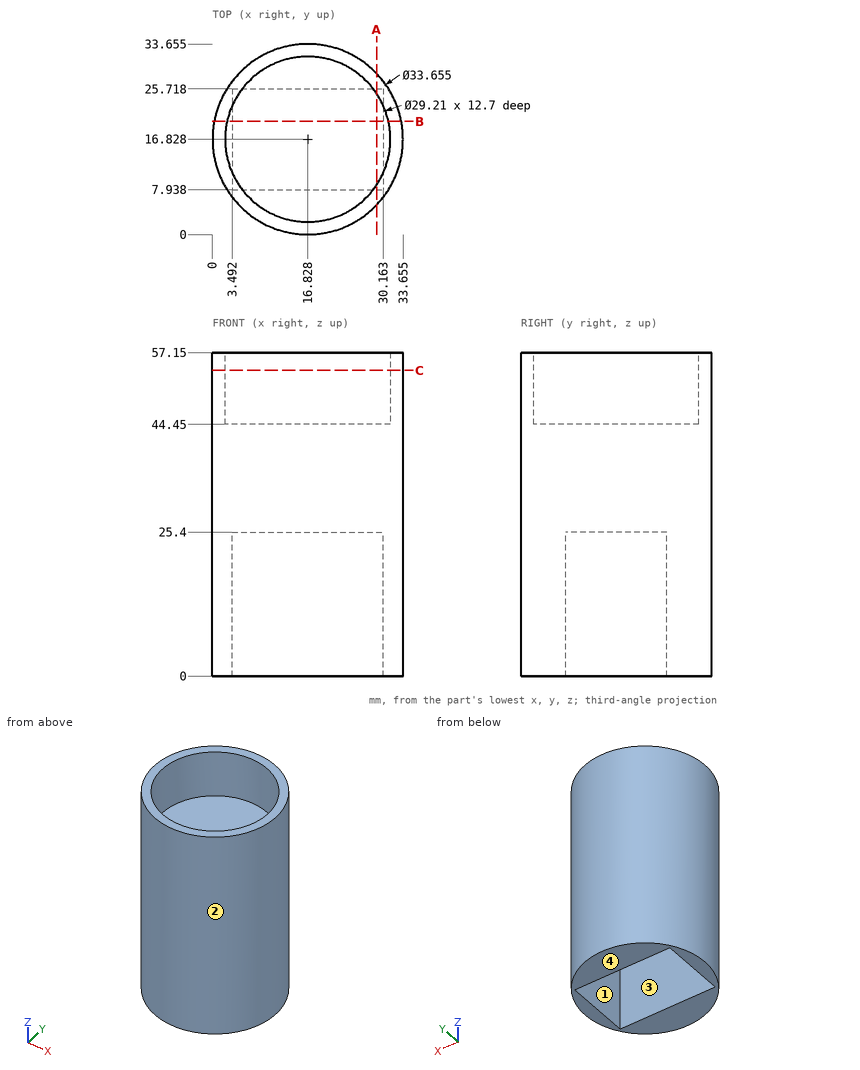
Print and shaded views of the part. All mm, measured from the part's lowest x, y and z. Round coordinates to 2 decimals unless told otherwise and drop trailing zeros. Write each loop counter-clockwise with the first axis right and the second up, starting at its lowest first coordinate (ties: lowest second). Pieces come first, ordered by that corner, then holes. Notation, with made-up numbers: (10.5, 53.25) - (24.5, 53.25) arc R17 cw to (24.5, 84.25) - close; hole circle Ø3 at (-32.5, -21). An arc over 180 degrees is marked (long way). One line per item, written item: value.
(1) Cut at B-B, the plane y = 20. Give the cut face in (x, z).
Values follow:
outline: (0.3, 0) - (3.49, 0) - (3.49, 25.4) - (30.16, 25.4) - (30.16, 0) - (33.35, 0) - (33.35, 57.15) - (31.08, 57.15) - (31.08, 44.45) - (2.57, 44.45) - (2.57, 57.15) - (0.3, 57.15) - close
(2) Drop flat-ended pins along their axis: P1, Ø5, axis at x = 5.5, z = 27, coming from the -Y side; P2, Ø19.5, axis at x = 13, y = 19.5, coming from the -Z side; P3, Ø9, axis at x = 23, y = 10.5, coming from the +Z side; P4, Ø1, axis at y = 10.5, z = 32, coming from the -X side. Give the stop position or say it passes through.
Values follow:
P1: stops at y = 2.5
P2: stops at z = 0
P3: stops at z = 44.45
P4: stops at x = 1.04
(3) Two-plate mould, pull along X, no slides. Class the marked faces 1, 2, 3 and 4: pulls with the +X half, pulls with the -X half, needs draft (parallel to the pull), parting line crosses it, or undercut.
Values follow:
face 1: undercut
face 2: parting line crosses it
face 3: undercut
face 4: needs draft
(4) Cut at C-C, the plane z = 54. Give the cut face in (x, y) (1 decimal).
Values follow:
outline: circle Ø33.7 at (16.8, 16.8); hole circle Ø29.2 at (16.8, 16.8)
(5) Wall check: probe 1 along X at (y, z) = (17, 3) (1 decimal); probe 2 along Z at (x, y) = (24, 17.5); probe 3 along Z at (x, y) = (31, 19). Give the ranges that are in metal, low to high.
Values follow:
probe 1: x = 0 to 3.5, 30.2 to 33.7
probe 2: z = 25.4 to 44.45
probe 3: z = 0 to 44.45
(6) Cut at A-A, the plane x = 29. Give the cut face in (y, z).
Values follow:
outline: (5.21, 0) - (7.94, 0) - (7.94, 25.4) - (25.72, 25.4) - (25.72, 0) - (28.45, 0) - (28.45, 57.15) - (24.9, 57.15) - (24.9, 44.45) - (8.76, 44.45) - (8.76, 57.15) - (5.21, 57.15) - close
